Autodesk Inventor part; units mm, degrees
ref_plane "Work Plane1" through (0, 2.3178, 0) normal (0, -1, 0) x (1, 0, 0)
ref_plane "Work Plane2" through (-5.5905, 0, -10.5766) normal (0, 0, 1) x (1, 0, 0)
ref_plane "YZ Plane" through (0, 0, 0) normal (1, 0, 0) x (0, 1, 0)
sketch "Sketch1" plane through (0, 0, 0) normal (0, 1, 0) x (-1, 0, 0)
  line L0 (0, 0) -> (7.7978, 0) construction
  line L1 (7.7978, 0) -> (7.7978, -21.1531) construction
  line L2 (7.7978, -21.1531) -> (0, -21.1531) construction
  line L3 (0, -21.1531) -> (0, 0) construction
  line L4 (7.7978, -10.5766) -> (7.7978, -2.7788) construction
  line L5 (7.7978, -2.7788) -> (0, -2.7788) construction
  line L6 (0, -2.7788) -> (0, -18.3744) construction
  line L7 (0, -18.3744) -> (7.7978, -18.3744) construction
  line L8 (7.7978, -18.3744) -> (7.7978, -2.7788) construction
  line L9 (7.7978, 0) -> (5.5905, 0) construction
  line L10 (5.5905, 0) -> (5.5905, -2.7788) construction
  line L11 (5.5905, -2.7788) -> (7.7978, -2.7788) construction
  line L12 (7.7978, -2.7788) -> (7.7978, 0) construction
  line L13 (7.7978, -10.5766) -> (0, -10.5766) construction
  line L14 (5.5905, -21.1531) -> (5.5905, -18.3744) construction
  line L15 (3.8989, 0) -> (3.8989, -21.1531) construction
  line L16 (2.2073, 0) -> (2.2073, -2.7788) construction
  line L17 (2.2073, -21.1531) -> (2.2073, -18.3744) construction
  line L18 (7.7978, 0) -> (7.7978, -21.1531)
  line L19 (7.7978, -21.1531) -> (5.5905, -21.1531)
  line L20 (5.5905, -21.1531) -> (5.5905, -18.3744)
  line L21 (5.5905, -18.3744) -> (2.2073, -18.3744)
  line L22 (2.2073, -18.3744) -> (2.2073, -21.1531)
  line L23 (2.2073, -21.1531) -> (0, -21.1531)
  line L24 (0, -21.1531) -> (0, 0)
  line L25 (0, 0) -> (2.2073, 0)
  line L26 (2.2073, 0) -> (2.2073, -2.7788)
  line L27 (2.2073, -2.7788) -> (5.5905, -2.7788)
  line L28 (5.5905, -2.7788) -> (5.5905, 0)
  line L29 (5.5905, 0) -> (7.7978, 0)
  dimension "d0" = 7.7978
  dimension "d1" = 21.1531
  dimension "d2" = 7.7978
  dimension "d3" = 7.7978
  dimension "d4" = 15.5956
  dimension "d5" = 2.2073
extrude "Extrusion1" add sketch "Sketch1" along normal blind 3.236
sketch "Sketch2" plane through (0, 3.236, 0) normal (0, 1, 0) x (1, 0, 0)
  line L0 (0, 0) -> (0, 21.1531) construction
  line L1 (0, 10.5766) -> (-7.7978, 10.5766) construction
  line L2 (-7.7978, 21.1531) -> (-7.7978, 0) construction
  line L3 (0, 10.5766) -> (-3.8989, 10.5766) construction
  line L4 (-3.8989, 10.5766) -> (-3.8989, 6.6777) construction
  line L5 (-3.8989, 6.6777) -> (0, 6.6777) construction
  line L6 (0, 6.6777) -> (0, 10.5766) construction
  circle A0 centre (-3.8989, 6.6777) radius 2.4498
  dimension "d8" = 3.8989
  dimension "d9" = 3.8989
  dimension "d10" = 4.8997
extrude "Extrusion2" add sketch "Sketch2" along normal blind 1.9837
pattern_linear "Rectangular Pattern1" count 2 spacing 7.7978 along (0, 0, -1) of "Extrusion2"
shell "Shell1" thickness 1.4732 removed faces 1 at (-3.335, 0, -7.9773)
sketch "Sketch3" plane through (-6.3246, 1.7628, -16.9012) normal (0, -1, 0) x (1, 0, 0)
  circle A0 centre (2.4257, 10.2235) radius 2.4498 construction
  circle A1 centre (2.4257, 2.4257) radius 2.4498 construction
  line L0 (2.4257, 10.2235) -> (2.4257, 2.4257) construction
  circle A2 centre (2.4257, 6.3246) radius 1.4491
  point P0 (6.3246, 16.9012)
extrude "Extrusion3" add sketch "Sketch3" along normal up to surface (1.7628 mm away)
ref_plane "Work Plane1" through (0, 2.3178, 0) normal (0, -1, 0) x (1, 0, 0)
sketch "Sketch5" plane through (0, 2.3178, 0) normal (0, -1, 0) x (1, 0, 0)
  line L0 (-7.7978, -21.1531) -> (-7.7978, 0) construction
  line L1 (-7.7978, 0) -> (-7.7978, 1.8186) construction
  line L2 (-7.7978, 0) -> (-5.9792, 0) construction
  line L3 (-7.7978, 1.8186) -> (0, 1.8186) construction
  line L4 (0, 1.8186) -> (0, 4.1377) construction
  line L5 (0, 4.1377) -> (-7.7978, 4.1377) construction
  line L6 (-7.7978, 4.1377) -> (-7.7978, 1.8186) construction
  line L7 (-7.7978, 4.1377) -> (-5.5905, 4.1377) construction
  line L8 (-7.7978, 4.1377) -> (-5.5905, 4.1377) construction
  line L9 (-5.5905, 4.1377) -> (-2.2073, 4.1377) construction
  line L10 (-2.2073, 4.1377) -> (-2.2073, 3.4366) construction
  line L11 (-2.2073, 3.4366) -> (-5.5905, 3.4366) construction
  line L12 (-5.5905, 3.4366) -> (-5.5905, 4.1377) construction
  line L13 (-7.7978, 1.8186) -> (0, 1.8186)
  line L14 (0, 1.8186) -> (0, 4.1377)
  line L15 (0, 4.1377) -> (-2.2073, 4.1377)
  line L16 (-2.2073, 4.1377) -> (-2.2073, 3.4366)
  line L17 (-2.2073, 3.4366) -> (-5.5905, 3.4366)
  line L18 (-5.5905, 3.4366) -> (-5.5905, 4.1377)
  line L19 (-5.5905, 4.1377) -> (-7.7978, 4.1377)
  line L20 (-7.7978, 4.1377) -> (-7.7978, 1.8186)
  dimension "d28" = 1.8186
  dimension "d29" = 90
  dimension "d30" = 7.7978
  dimension "d31" = 2.319
  dimension "d32" = 2.2073
  dimension "d33" = 0
  dimension "d34" = 3.3833
  dimension "d35" = 0.701
revolve "Revolution1" add sketch "Sketch5" angle 360 about axis through (-7.7978, 2.3178, 1.8186) along (1, 0, 0)
sketch "Sketch6" plane through (-2.2073, 0, 0) normal (0, 0, 1) x (1, 0, 0)
  line L0 (2.2073, 0) -> (0, 0)
  line L1 (0, 0) -> (0, 3.236)
  line L2 (2.2073, 0) -> (0, 0)
  line L3 (0, 0) -> (0, 3.236)
  line L4 (0, 3.236) -> (2.2073, 3.236)
  line L5 (2.2073, 3.236) -> (2.2073, 0)
  line L6 (-3.3833, 0) -> (-5.5905, 0)
  line L7 (-3.3833, 0) -> (-3.3833, 3.236)
  line L8 (-5.5905, 0) -> (-3.3833, 0)
  line L9 (-3.3833, 0) -> (-3.3833, 3.236)
  line L10 (-3.3833, 3.236) -> (-5.5905, 3.236)
  line L11 (-5.5905, 3.236) -> (-5.5905, 0)
extrude "Extrusion4" add sketch "Sketch6" along normal up to surface
ref_plane "Work Plane2" through (-5.5905, 0, -10.5766) normal (0, 0, 1) x (1, 0, 0)
mirror "Mirror1" about plane through (-5.5905, 0, -10.5766) normal (0, 0, 1) of "Revolution1", "Extrusion4"
properties part number "Weird circle things" material "ABS Plastic"
Geometry: final body of the model. Coordinates: model frame, mm. A direction names the side the tool comes from. Round coordinates to 2 decimals unless told otherwise and drop trailing zeros. Loops run counter-clockwise (first coordinate to the right, second up) from the corner with the lowest first, then second, coordinate; pieces in that order, holes last.
Q1. Section C-C on x = -4.25. State how many separate pieces and enclosed holes the cut face has, plus the area to 3 significant figures.
Q2. Section D-D on y = 2.7. Return loops of the section in (x, z).
Q3. Section A-A on y = 1.15. Return loops of the section in (x, z).
Q4. Pin query (flat end, axial travel): P1, Ø2.5, axis at x = -3.9, z = -14.48, coming from the -Y side; P2, Ø1.4, axis at x = -3, y = 0.5, coming from the +Z side; P3, Ø1.6, axis at x = -3.5, y = 1, coming from the -Z side. Return the tip coordinate at first contact, or that it passes through.
Q5. Material intervals for L1, parallel to X at y = 1.55, z = -16.75; L2, parallel to X at y = 2.8, z = -19.5; L3, parallel to Z at x = -4.25, y = 2, sorted ascending.
Q6. Access query for faces 3 (the cylindrical face through (-1.119, 3.5, 3.814)), 4 (the cylindrical face through (-3.923, 0.738, 1.468)), 5 (the flat face through (-4, 2, -2.779)), 6 (the cylindrical face through (-4.43, 4.21, -9.07)), 7 (the flat face through (-6.325, 1, -10)). Directions: +Z, -Z, +X, -X, +Y, -Y. A direction counts if a zero-diameter tool reaches every point of the face in a straight line with its end or side. Return the directions, or none.
Q7. Section B-B on z = -18.75. Return loops of the section in (x, y), plus the area to 3 significant figures.
Q8. Pull-direction query (Z, two-part tool) for faces 1 (the flat face through (-4, 5.22, -7)), 2 (the flat face through (-4, 3.236, -10)); classes: released by +Z, released by -Z, zero draft, split by the parting line, or undercut.
Evaluation:
1. separate pieces: 3
1. enclosed holes: 0
1. area: 61.6 mm2
2. outline: (-7.8, -25.26) - (-5.59, -25.26) - (-5.59, -24.54) - (-2.21, -24.54) - (-2.21, -25.26) - (0, -25.26) - (0, 4.11) - (-2.21, 4.11) - (-2.21, 3.39) - (-5.59, 3.39) - (-5.59, 4.11) - (-7.8, 4.11) - close; hole (-5.59, -21.4) - (-2.21, -21.4) - (-2.21, -18.37) - (-5.59, -18.37) - close; hole (-5.59, -2.78) - (-2.21, -2.78) - (-2.21, 0.25) - (-5.59, 0.25) - close; hole circle Ø1.95 at (-3.9, -14.48); hole circle Ø1.95 at (-3.9, -6.68)
3. outline: (-7.8, -24.98) - (-5.59, -24.98) - (-5.59, -24.09) - (-2.21, -24.09) - (-2.21, -24.98) - (0, -24.98) - (0, 3.82) - (-2.21, 3.82) - (-2.21, 2.94) - (-5.59, 2.94) - (-5.59, 3.82) - (-7.8, 3.82) - close; circle Ø2.9 at (-3.9, -10.58); hole (-6.32, -16.9) - (-1.47, -16.9) - (-1.47, -4.25) - (-6.32, -4.25) - close; hole (-5.59, -21.85) - (-2.21, -21.85) - (-2.21, -18.37) - (-5.59, -18.37) - close; hole (-5.59, -2.78) - (-2.21, -2.78) - (-2.21, 0.7) - (-5.59, 0.7) - close
4. P1: stops at y = 1.76
4. P2: stops at z = 2.99
4. P3: stops at z = -24.5
5. L1: x = -7.8 to -6.32, -1.47 to 0
5. L2: x = -7.8 to -5.59, -2.21 to 0
5. L3: z = -24.56 to -21.39, -18.37 to -15.39, -13.56 to -7.59, -5.77 to -2.78, 0.23 to 3.41
6. face 3: +X, -X
6. face 4: none
6. face 5: +Y, -Y
6. face 6: +Y
6. face 7: -Y
7. outline: (-7.8, 0) - (-5.59, 0) - (-5.59, 3.24) - (-7.8, 3.24) - close; (-2.21, 0) - (0, 0) - (0, 3.24) - (-2.21, 3.24) - close
7. area: 14.3 mm2
8. face 1: zero draft
8. face 2: undercut
